from build123d import *

# Parameters (mm, degrees)
SKETCH1_R                       = 58.299985
BOSS_EXTRUDE1_DEPTH             = 1370.16998
SKETCH2_R                       = 57.15
CUT_EXTRUDE1_DEPTH              = 1370.16998
SKETCH3_W                       = 3
SKETCH3_H                       = 300
CUT_EXTRUDE2_DEPTH              = 10
CIRPATTERN1_COUNT               = 3
F_6_0_204_DIAMETER_HOLE1_REACH  = 1378.358
F_6_0_204_DIAMETER_HOLE1_BORE_R = 2.5908
CIRPATTERN2_COUNT               = 5


with BuildPart() as part:
    # Sketch1 → Boss-Extrude1 (new body)
    with BuildSketch(Plane(origin=(0, 0, 0), x_dir=(1, 0, 0), z_dir=(0, 1, 0))):
        with Locations(Location((0, 0, 0), (0, 0, 270))):
            Circle(SKETCH1_R)
    extrude(amount=BOSS_EXTRUDE1_DEPTH)

    # Sketch2 → Cut-Extrude1 (cut)
    with BuildSketch(Plane(origin=(0, 0, 0), x_dir=(1, 0, 0), z_dir=(0, 1, 0))):
        with Locations(Location((0, 0, 0), (0, 0, 270))):
            Circle(SKETCH2_R)
    extrude(amount=CUT_EXTRUDE1_DEPTH, mode=Mode.SUBTRACT)

    # Sketch3 → Cut-Extrude2 (cut)
    with BuildSketch(Plane(origin=(58.299985, 0, 0), x_dir=(0, 0, -1), z_dir=(1, 0, 0))):
        with Locations((0, 150)):
            Rectangle(SKETCH3_W, SKETCH3_H)
    cut_extrude2 = extrude(amount=-CUT_EXTRUDE2_DEPTH, mode=Mode.SUBTRACT)

    # CirPattern1: Cut-Extrude2 ×3 about axis
    cirpattern1_axis = Axis((0, 0, 0), (0, 1, 0))
    for i in range(1, CIRPATTERN1_COUNT):
        add(cut_extrude2.rotate(cirpattern1_axis, i * 360 / CIRPATTERN1_COUNT), mode=Mode.SUBTRACT)

    # 6 _0.204_ Diameter Hole1 bore → 6 _0.204_ Diameter Hole1 (cut, up to next)
    with BuildSketch(Plane(origin=(58.299985, 0, 0), x_dir=(0, 0, -1), z_dir=(1, 0, 0)), mode=Mode.PRIVATE) as f_6_0_204_diameter_hole1_sk1:
        with Locations((0, 1353.17738)):
            Circle(F_6_0_204_DIAMETER_HOLE1_BORE_R)
    f_6_0_204_diameter_hole1_tool1 = extrude(f_6_0_204_diameter_hole1_sk1.sketch, amount=-F_6_0_204_DIAMETER_HOLE1_REACH, mode=Mode.PRIVATE) & part.part
    # 6 _0.204_ Diameter Hole1 bore → 6 _0.204_ Diameter Hole1 (cut, up to next)
    with BuildSketch(Plane(origin=(58.299985, 0, 0), x_dir=(0, 0, -1), z_dir=(1, 0, 0)), mode=Mode.PRIVATE) as f_6_0_204_diameter_hole1_sk2:
        with Locations((0, 1273.16738)):
            Circle(F_6_0_204_DIAMETER_HOLE1_BORE_R)
    f_6_0_204_diameter_hole1_tool2 = extrude(f_6_0_204_diameter_hole1_sk2.sketch, amount=-F_6_0_204_DIAMETER_HOLE1_REACH, mode=Mode.PRIVATE) & part.part
    f_6_0_204_diameter_hole1_1 = f_6_0_204_diameter_hole1_tool1.solids().sort_by_distance((58.299985, 1353.17738, 0))[0]
    add(f_6_0_204_diameter_hole1_1, mode=Mode.SUBTRACT)
    f_6_0_204_diameter_hole1_2 = f_6_0_204_diameter_hole1_tool2.solids().sort_by_distance((58.299985, 1273.16738, 0))[0]
    add(f_6_0_204_diameter_hole1_2, mode=Mode.SUBTRACT)
    f_6_0_204_diameter_hole1 = f_6_0_204_diameter_hole1_1 + f_6_0_204_diameter_hole1_2  # 6 _0.204_ Diameter Hole1 as one shape, for the pattern or mirror that repeats it

    # CirPattern2: 6 _0.204_ Diameter Hole1 ×5 about axis
    cirpattern2_axis = Axis((0, 0, 0), (0, -1, 0))
    for i in range(1, CIRPATTERN2_COUNT):
        add(f_6_0_204_diameter_hole1.rotate(cirpattern2_axis, i * 360 / CIRPATTERN2_COUNT), mode=Mode.SUBTRACT)


solid = part.part
Verification items for the finished model (mm, model axes). Give positions to 0.01 mm unless a question says otherwise; leave off trailing zeros. Loops run counter-clockwise (first coordinate to the right, second up) from the corner with the lowest first, then second, coordinate; pieces in that order, holes last.
1) Sectioned sample at C-C, the plane y = 810. Enter the section's corners in (x, z), then the cut area to 3 significant figures.
2) Draft check along X on faces 1 (the cylindrical face through (2.513, 675.494, -57.095)), 2 (the flat face through (-43, 1370.17, 39)), 3 (the cylindrical face through (57.804, 675.494, -7.589)). Enter one of: pulls with the +X half, pulls with the -X half, needs draft (parallel to the pull), parting line crosses it, or undercut.
3) Sectioned sample at A-A, the plane y = 102.5. Enter the section's corners in (x, z), then the cut area to 3 significant figures.
4) Thickness scan on line 1 along Y through (x, z) = (57.8, 0); line 2 along X through (y, z) = (128, -3); line 3 along X through (y, z) = (795, 0.5). Record the ranges inside material, lowest first.
5) Depth check by flat-ended pin: pin 1 Ø1.2 at (x, z) = (-28.5, 49.5) entering from -Y; pin 2 Ø6.5 at (y, z) = (1273.17, 0) entering from -X; pin 3 Ø6 at (y, z) = (220.5, 24) entering from -X; pin 4 Ø8 at (x, z) = (-37, 36) entering from +Y. Enter the tip coordinate at first touch or a pass-through.
6) Sectioned sample at B-B, the plane x = 0. Enter the section's corners in (y, z), then the cut area to 3 significant figures.
Answers:
1. outline: circle Ø116.6 at (0, 0); hole circle Ø114.3 at (0, 0)
1. area: 417 mm2
2. face 1: undercut
2. face 2: needs draft
2. face 3: parting line crosses it
3. outline: (-30.44, -49.72) - (-29.86, -48.73) arc R57.15 cw to (-29.86, 48.73) - (-30.44, 49.72) arc R58.3 ccw to start; (-27.84, -51.22) arc R58.3 ccw to (58.28, -1.5) - (57.13, -1.5) arc R57.15 cw to (-27.27, -50.23) - close; (-27.84, 51.22) - (-27.27, 50.23) arc R57.15 cw to (57.13, 1.5) - (58.28, 1.5) arc R58.3 ccw to start
3. area: 407 mm2
4. line 1: y = 300 to 1270.58, 1275.76 to 1350.59, 1355.77 to 1370.17
4. line 2: x = -58.22 to -57.07, 57.07 to 58.22
4. line 3: x = -58.3 to -57.15, 57.15 to 58.3
5. pin 1: stops at y = 300
5. pin 2: stops at x = -58.3
5. pin 3: stops at x = -54.39
5. pin 4: passes through
6. outline: (0, -58.3) - (1370.17, -58.3) - (1370.17, -57.15) - (0, -57.15) - close; (0, 57.15) - (1370.17, 57.15) - (1370.17, 58.3) - (0, 58.3) - close
6. area: 3,150 mm2
